from build123d import *

# Parameters (mm, degrees)
SKETCH_W        = 60
SKETCH_H        = 13
PAD_DEPTH       = 13
POCKET_DEPTH    = 16
SKETCH002_W     = 31.5
SKETCH002_H     = 18.692561
POCKET001_DEPTH = 10
SKETCH003_W     = 18
SKETCH003_H     = 8
POCKET002_DEPTH = 5


with BuildPart() as part:
    # Sketch → Pad (new body)
    with BuildSketch(Plane.XY):
        with Locations((0, 6.5)):
            Rectangle(SKETCH_W, SKETCH_H)
    extrude(amount=PAD_DEPTH)

    # Sketch001 (on Face3 of Pad) → Pocket (cut)
    with BuildSketch(Plane.XZ):
        Polygon((-33.208946, 6), (-18.5, 6), (-18.5, 16.342094), (18.5, 16.342094), (18.5, 6), (35.755672, 6), (31.923449, 22.090439), (-34.230431, 22.090439), align=None)
    extrude(amount=-POCKET_DEPTH, mode=Mode.SUBTRACT)

    # Sketch002 (on Face10 of Pocket) → Pocket001 (cut)
    with BuildSketch(Plane.XZ):
        with Locations((0, 0.65372)):
            Rectangle(SKETCH002_W, SKETCH002_H)
    extrude(amount=-POCKET001_DEPTH, mode=Mode.SUBTRACT)

    # Sketch003 (on Face12 of Pocket001) → Pocket002 (cut)
    with BuildSketch(Plane.XZ.offset(-10)):
        with Locations((0, 6.183331)):
            Rectangle(SKETCH003_W, SKETCH003_H)
    extrude(amount=-POCKET002_DEPTH, mode=Mode.SUBTRACT)


solid = part.part
Geometry check sheet. Reference: the model listing, model coordinates, mm. A direction names the side the tool comes from. Round coordinates to 2 decimals unless told otherwise and drop trailing zeros. Write each loop counter-clockwise with the first axis right and the second up, starting at its lowest first coordinate (ties: lowest second). Pieces come first, ordered by that corner, then holes. Notation, with made-up numbers: (85, -30) -> (103, -30) arc R22 ccw to (103, 4) -> close; hole circle Ø5 at (79, -11). An arc over 180 degrees is marked (long way). One line per item, written item: value. Start each with the question number.
(1) Draft check along Z on faces 6 (the flat face through (0, 11, 0)), 7 (the flat face through (0, 11, 2.183)), 8 (the flat face through (-18.5, 6, 9)). Enter one of: +Z half, -Z half, draft (parallel to the pull), parting line (faces both ways), or undercut.
(2) Scan lines: line 1 (Z direction, x = 8, y = 11.25); line 2 (X direction, y = 6.5, z = 4); line 3 (X direction, y = 10.5, z = 9.25). Record each from-to range of solid material in increasing order. Write a range as [from, to].
(3) Cross-section at A-A, the plane z = 9.25. Record the cut outline in (x, y), and give its area (3 significant figures).
(4) Cross-section at C-C, the plane y = 1.25. Record the cut outline in (x, z).
(5) Cross-section at B-B, the plane x = 3.5. Record the cut outline in (y, z).
(6) Go/stop test with flat-tipped pins: pin 1 Ø3.5 at (x, y) = (-24, 7.5) entering from +Z; pin 2 Ø2.5 at (x, y) = (-1, 12) entering from -Z; pin 3 Ø3 at (x, z) = (-7.5, 3.5) entering from -Y; pin 4 Ø1.5 at (y, z) = (10, 9.5) entering from -X. Record where each tip stops, or that it passes through.
(7) Access from +Z, -Z, +X, -X, +Y, -Y to the whole of each face (thin tool, end or side, straight path). Record for faces 1 (the flat face through (15.75, 5, 5)), 2 (the flat face through (30, 6, 3)), 3 (the flat face through (24, 6, 6)), 4 (the flat face through (0, 11, 10.183)), 5 (the flat face through (-24, 6, 6)).
(8) Cross-section at D-D, the plane z = 1. Record the cut outline in (x, y).
Answer:
1. face 6: -Z half
1. face 7: undercut
1. face 8: draft
2. line 1: [0, 2.18], [10.18, 13]
2. line 2: [-30, -15.75], [15.75, 30]
2. line 3: [-18.5, -9], [9, 18.5]
3. outline: (-18.5, 0) -> (-15.75, 0) -> (-15.75, 10) -> (-9, 10) -> (-9, 13) -> (-18.5, 13) -> close; (9, 10) -> (15.75, 10) -> (15.75, 0) -> (18.5, 0) -> (18.5, 13) -> (9, 13) -> close
3. area: 112 mm²
4. outline: (-30, 0) -> (-15.75, 0) -> (-15.75, 10) -> (15.75, 10) -> (15.75, 0) -> (30, 0) -> (30, 6) -> (18.5, 6) -> (18.5, 13) -> (-18.5, 13) -> (-18.5, 6) -> (-30, 6) -> close
5. outline: (0, 10) -> (10, 10) -> (10, 10.18) -> (13, 10.18) -> (13, 13) -> (0, 13) -> close; (10, 0) -> (13, 0) -> (13, 2.18) -> (10, 2.18) -> close
6. pin 1: z = 6
6. pin 2: z = 0
6. pin 3: y = 10
6. pin 4: x = -18.5
7. face 1: -Z, -Y
7. face 2: +Z, -Z, +X, +Y, -Y
7. face 3: +Z, +X, +Y, -Y
7. face 4: +Y
7. face 5: +Z, -X, +Y, -Y
8. outline: (-30, 0) -> (-15.75, 0) -> (-15.75, 10) -> (15.75, 10) -> (15.75, 0) -> (30, 0) -> (30, 13) -> (-30, 13) -> close
